Here's the drawing with two shaded views (mm, measured from the low corner). I have some questions. Coordinates: 2 decimals unless noted, no trailing zeros. Write each loop counter-clockwise with the first axis right and the second up, starting at its lowest first coordinate (ties: lowest second). Pieces come first, ordered by that corner, then holes.
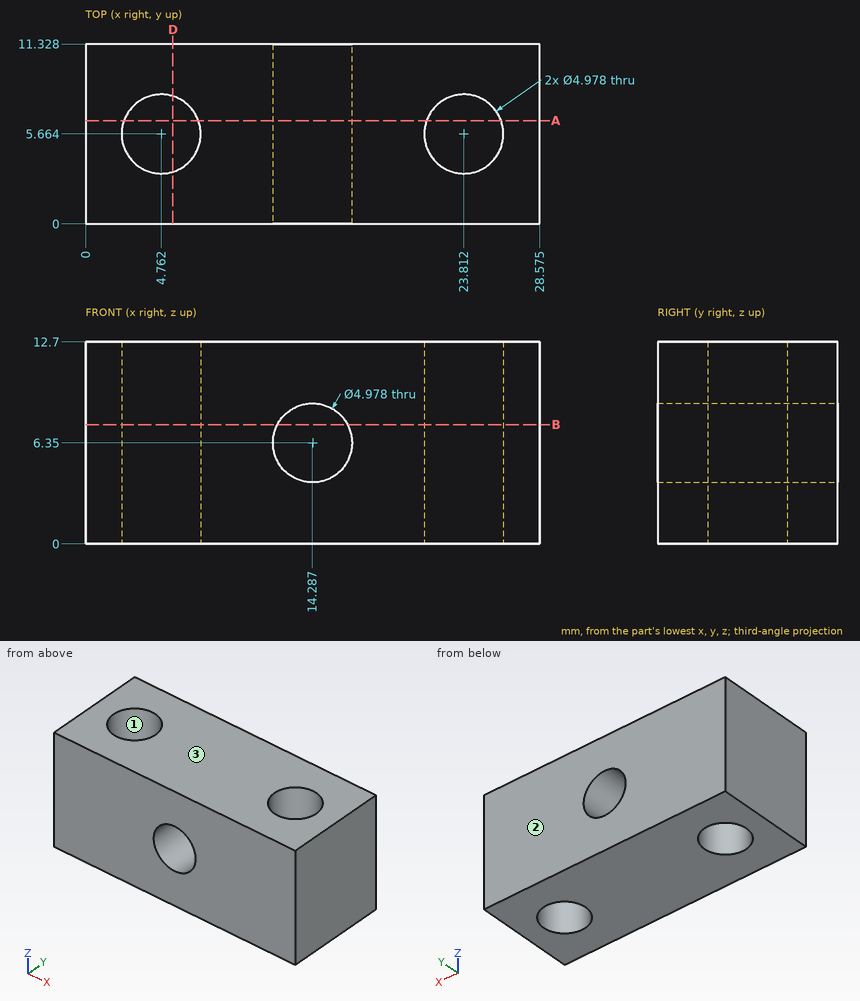
1. I want a section at B-B on z = 7.5. Please give me the cut outline in (x, y) (1 decimal).
Verdict:
outline: (0, 0) - (12.1, 0) - (12.1, 11.3) - (0, 11.3) - close; (16.5, 0) - (28.6, 0) - (28.6, 11.3) - (16.5, 11.3) - close; hole circle Ø5 at (4.8, 5.7); hole circle Ø5 at (23.8, 5.7)
2. I want a section at A-A on y = 6.5. Give the number of separate pieces and of enclosed holes in the cut face, plus the area to 3 significant figures.
Verdict:
separate pieces: 3
enclosed holes: 1
area: 224 mm2
3. I want a section at D-D on x = 5.5. Please give me the cut outline in (y, z).
Verdict:
outline: (0, 0) - (3.29, 0) - (3.29, 12.7) - (0, 12.7) - close; (8.04, 0) - (11.33, 0) - (11.33, 12.7) - (8.04, 12.7) - close
4. If we mould it in two halves opening along Y, with no side actions, what happens to the marked faces 1, 2 and 3? For each: pulls with the +Y half, pulls with the -Y half, needs draft (parallel to the pull), parting line crosses it, or undercut.
Verdict:
face 1: undercut
face 2: pulls with the +Y half
face 3: needs draft
5. Please list where these lines run through material, in increasing order: line 1 along Y through (x, z) = (23.75, 4) (1 decimal); line 2 along X through (y, z) = (6.5, 11) (1 decimal); line 3 along Z through (x, y) = (13.25, 3).
Verdict:
line 1: y = 0 to 3.2, 8.2 to 11.3
line 2: x = 0 to 2.4, 7.1 to 21.5, 26.2 to 28.6
line 3: z = 0 to 4.09, 8.61 to 12.7
6. For pin 1 (6.5 mm diameter, centred on x = 23.81, y = 5.66, fed in from -Z), with a flat end and sliding along its axis, tell me the tip position at first contact or that it passes through.
Verdict:
pin 1: stops at z = 0
